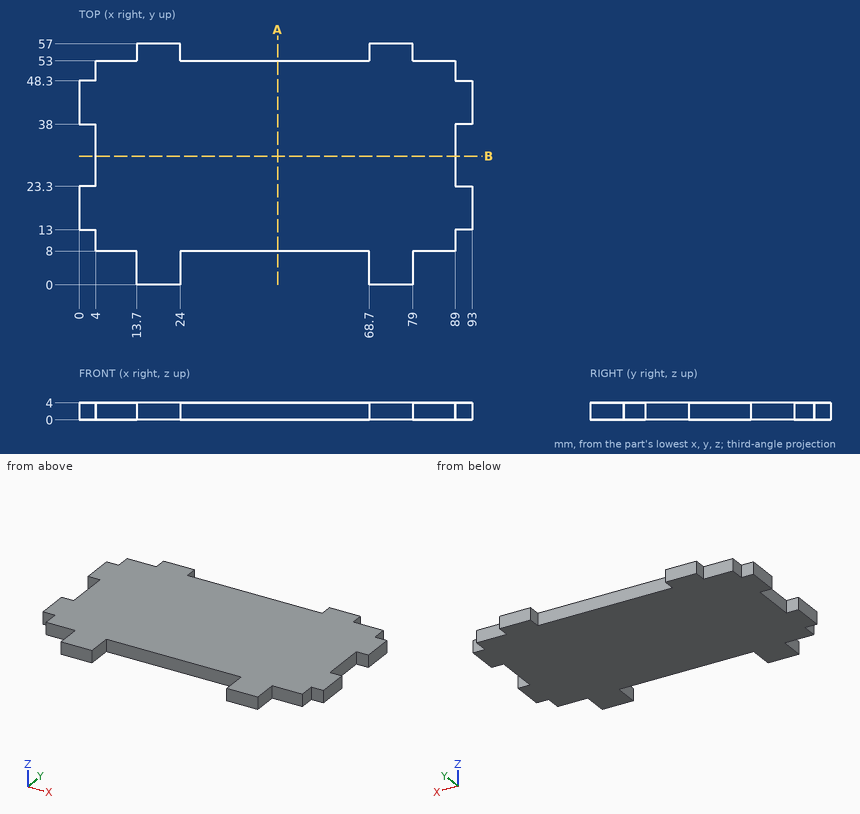
Verification items for this drawing (mm, ordinates from the low corner). Coordinates: 2 decimals unless noted, no trailing zeros. Loops run counter-clockwise (first coordinate to the right, second up) from the corner with the lowest first, then second, coordinate; pieces in that order, holes last. Notation, with made-up numbers: (-4.75, 82) - (43.25, 82) arc R14 cw to (43.25, 92) - close; hole circle Ø6 at (61, 23.25). An arc over 180 degrees is marked (long way). Use one line per item in the form item = value. Start each with the question number.
Item 1: Thickness scan on probe 1 along X at (y, z) = (5.5, 1.8); probe 2 along Y at (x, z) = (43, 1.55); probe 3 along X at (y, z) = (31, 3.35). Record the ranges inside material, lowest first.
Item 2: Gauge pin test, flat ends, axial feed: pin 1 (1.2 mm diameter, centred on x = 85.5, z = 2.5, fed in from -Y); pin 2 (1.2 mm diameter, centred on y = 51, z = 2, fed in from -X). Record the tip position at first contact, or that the pin passes through.
Item 3: Section check A-A, the plane x = 47. Enter the section's corners in (y, z).
Item 4: Section check B-B, the plane y = 30.5. Enter the section's corners in (x, z).
Computed:
q1.probe_1 = 13.7 to 24, 68.7 to 79
q1.probe_2 = 8 to 53
q1.probe_3 = 4 to 89
q2.pin_1 = 8
q2.pin_2 = 4
q3.outline = (8, 0) - (53, 0) - (53, 4) - (8, 4) - close
q4.outline = (4, 0) - (89, 0) - (89, 4) - (4, 4) - close
